from build123d import *

# Parameters (mm, degrees)
CROQUIS1_R              = 10
SALIENTE_EXTRUIR1_DEPTH = 25
CORTAR_EXTRUIR1_REACH   = 30.723
CROQUIS3_R              = 3.5
CROQUIS5_R              = 3.5
CROQUIS5_R_2            = 2
CORTAR_EXTRUIR3_DEPTH   = 34.541019662
CORTAR_EXTRUIR4_REACH   = 30.723
CROQUIS6_W              = 9.7
CROQUIS6_H              = 3.7
CROQUIS7_R              = 3.5
CORTAR_EXTRUIR5_DEPTH   = 3


with BuildPart() as part:
    # Croquis1 → Saliente-Extruir1 (new body)
    with BuildSketch(Plane(origin=(0, 0, 0), x_dir=(1, 0, 0), z_dir=(0, 1, 0))):
        with Locations(Location((0, 0, 0), (0, 0, 270))):
            Circle(CROQUIS1_R)
    extrude(amount=SALIENTE_EXTRUIR1_DEPTH)

    # Croquis3 → Cortar-Extruir1 (cut, up to next)
    with BuildSketch(Plane(origin=(0, 25, 0), x_dir=(1, 0, 0), z_dir=(0, 1, 0)), mode=Mode.PRIVATE) as cortar_extruir1_sk1:
        with Locations(Location((0, -4, 0), (0, 0, 270))):
            Circle(CROQUIS3_R)
    cortar_extruir1_tool1 = extrude(cortar_extruir1_sk1.sketch, amount=-CORTAR_EXTRUIR1_REACH, mode=Mode.PRIVATE) & part.part
    add(cortar_extruir1_tool1.solids().sort_by_distance((0, 25, 4))[0], mode=Mode.SUBTRACT)

    # Croquis5 → Cortar-Extruir3 (cut, through all)
    with BuildSketch(Plane(origin=(0, 0, -10), x_dir=(-1, 0, 0), z_dir=(0, 0, -1))):
        with Locations((0, 6)):
            Circle(CROQUIS5_R)
        with Locations((0, 20)):
            Circle(CROQUIS5_R_2)
    extrude(amount=-CORTAR_EXTRUIR3_DEPTH, mode=Mode.SUBTRACT)

    # Croquis6 → Cortar-Extruir4 (cut, up to next)
    with BuildSketch(Plane.XZ, mode=Mode.PRIVATE) as cortar_extruir4_sk1:
        with Locations((0, -3.15)):
            Rectangle(CROQUIS6_W, CROQUIS6_H)
    cortar_extruir4_tool1 = extrude(cortar_extruir4_sk1.sketch, amount=-CORTAR_EXTRUIR4_REACH, mode=Mode.PRIVATE) & part.part
    add(cortar_extruir4_tool1.solids().sort_by_distance((0, 0, -3.15))[0], mode=Mode.SUBTRACT)

    # Croquis7 → Cortar-Extruir5 (cut)
    with BuildSketch(Plane(origin=(0, 0, -10), x_dir=(-1, 0, 0), z_dir=(0, 0, -1))):
        with Locations((0, 20)):
            Circle(CROQUIS7_R)
    extrude(amount=-CORTAR_EXTRUIR5_DEPTH, mode=Mode.SUBTRACT)


solid = part.part
The model under review builds one solid part; all positions refer to its coordinate system, in mm. A direction names the side the tool comes from. Round coordinates to 2 decimals unless told otherwise and drop trailing zeros. Loops run counter-clockwise (first coordinate to the right, second up) from the corner with the lowest first, then second, coordinate; pieces in that order, holes last. Notation, with made-up numbers: (-16.75, 53.25) -> (29.25, 53.25) arc R13 ccw to (29.25, 74.25) -> close; hole circle Ø9 at (-2, -21). An arc over 180 degrees is marked (long way). Return JSON: item names as keys, results as strings.
(1) Add section B-B on z = -2.5. Write out the cut boundary in (x, y).
Solved:
{"outline": "(-9.68, 0) -> (-4.85, 0) -> (-4.85, 25) -> (-9.68, 25) -> close; (4.85, 0) -> (9.68, 0) -> (9.68, 25) -> (4.85, 25) -> close"}
(2) For faces 1 (the cylindrical face through (-1.908, 20.601, -0.373)), 2 (the flat face through (-2, 18, -7)), 3 (the flat face through (-4.85, 12, -3)), list the 3-axis set-ups (+Z, -Z, +X, -X, +Y, -Y) from which the entire face can be reached by the end or side of a thin tool; tool diameter is ignored.
Solved:
{"face 1": "+Z, -Z", "face 2": "-Z", "face 3": "+Y, -Y"}
(3) The part is to be moulded in two halves that separate along Y. For faces 4 (the flat face through (0, 25, 0)), 5 (the flat face through (0, 12, -5)), 6 (the cylindrical face through (0, 22, -6)), say which applies: released by +Y, released by -Y, zero draft, split by the parting line, or undercut.
Solved:
{"face 4": "released by +Y", "face 5": "zero draft", "face 6": "undercut"}
(4) Add section D-D on y = 11.5. Write out the cut boundary in (x, z).
Solved:
{"outline": "circle Ø20 at (0, 0); hole (-4.85, -5) -> (4.85, -5) -> (4.85, -1.3) -> (-4.85, -1.3) -> close; hole circle Ø7 at (0, 4)"}
(5) Add section A-A on y = 21.5. Write out the cut boundary in (x, z).
Solved:
{"outline": "(-4.85, -5) -> (-4.85, -1.3) -> (-1.32, -1.3) -> (-1.32, 0.76) arc R3.5 cw to (-1.32, 7.24) -> (-1.32, 9.91) arc R10 ccw to (-3.16, -9.49) -> (-3.16, -7) -> (-1.32, -7) -> (-1.32, -5) -> close; (1.32, -7) -> (3.16, -7) -> (3.16, -9.49) arc R10 ccw to (1.32, 9.91) -> (1.32, 7.24) arc R3.5 cw to (1.32, 0.76) -> (1.32, -1.3) -> (4.85, -1.3) -> (4.85, -5) -> (1.32, -5) -> close"}
(6) Add section C-C on x = 0. State how many separate pieces and enclosed holes the cut face has, plus the area to 3 significant figures.
Solved:
{"separate pieces": "9", "enclosed holes": "0", "area": "121 mm2"}
(7) For pin 1 (3 mm diameter, centred on y = 17, z = -2, fed in from +X); pin 2 (4 mm diameter, centred on y = 14.5, z = -4, fed in from +X); pin 3 (6.5 mm diameter, centred on x = 0, z = 4, fed in from -Y); pin 4 (12 mm diameter, centred on x = -6.5, y = 17, fed in from +Z), all flat-tipped, find the tip position at first contact; note any pin that passes through.
Solved:
{"pin 1": "x = 9.99", "pin 2": "x = 9.8", "pin 3": "through", "pin 4": "z = 9.99"}
(8) For line 1 (Y direction, x = 0, z = -0.5); line 2 (Z direction, x = 0, y = 16.25); line 3 (Y direction, x = 0, z = -7.5), list the stretches that pass through material, from the lowest coordinate up.
Solved:
{"line 1": "0 to 2.5, 9.5 to 18, 22 to 25", "line 2": "-10 to -5, -1.3 to 0.5, 7.5 to 10", "line 3": "0 to 2.5, 9.5 to 16.5, 23.5 to 25"}
